```python
from build123d import *

# Parameters (mm, degrees)
CLAMP_START                     = -20.15
CLAMP_X_BASE_DEPTH              = 37.1
WIRE_START                      = -4.99
WIRE_CHANNEL_X_BASE_Z_5_0_DEPTH = 3.42
WIRE_START_2                    = -4.84
SKETCH3_W                       = 1.6
SKETCH3_H                       = 4.320657937
WIRE_NOTCH_X_BASE_Z_5_0_DEPTH   = 3.12
EAR_START                       = -26.1
SKETCH4_W                       = 4.582851153
SKETCH4_H                       = 2.45
EAR_X_BASE_26_DEPTH             = 5.95
EAR_START_2                     = 16.95
SKETCH5_W                       = 4.582851153
SKETCH5_H                       = 2.45
EAR_X_BASE_17_DEPTH             = 5.95
CUT_EXTRUDE3_START              = -6.55
SKETCH6_R                       = 1.05
CUT_EXTRUDE3_DEPTH              = 2.65
CUT_EXTRUDE4_START              = -5.91
SKETCH7_R                       = 2
CUT_EXTRUDE4_DEPTH              = 1.92
CUT_EXTRUDE5_START              = -5.91
SKETCH8_W                       = 2.082851153
SKETCH8_H                       = 4
CUT_EXTRUDE5_DEPTH              = 1.92
CUT_EXTRUDE6_START              = -5.91
CUT_EXTRUDE6_DEPTH              = 1.92
CUT_EXTRUDE7_START              = -5.91
CUT_EXTRUDE7_DEPTH              = 1.92
BOSS_EXTRUDE4_START             = -4
SKETCH11_W                      = 3.882851153
SKETCH11_H                      = 7.3
BOSS_EXTRUDE4_DEPTH             = 0.75


with BuildPart() as part:
    # Sketch1 → Clamp +X base (new body)
    with BuildSketch(Plane.XY.offset(CLAMP_START)):
        Polygon((13.367148847, -4), (17.397275866, -4), (17.397275866, -8.470102587), (13.367148847, -10.796897507), align=None)
    extrude(amount=CLAMP_X_BASE_DEPTH)

    # Sketch2 → Wire channel +X base Z -5.0 (cut)
    with BuildSketch(Plane.XY.offset(WIRE_START)):
        Polygon((11.102085338, -12.220102587), (19.762339376, -7.220102587), (18.912339376, -5.747859401), (10.252085338, -10.747859401), align=None)
    extrude(amount=WIRE_CHANNEL_X_BASE_Z_5_0_DEPTH, mode=Mode.SUBTRACT)

    # Sketch3 → Wire notch +X base Z -5.0 (cut)
    with BuildSketch(Plane.XY.offset(WIRE_START_2)):
        with Locations((16.897275866, -6.060328969)):
            Rectangle(SKETCH3_W, SKETCH3_H)
    extrude(amount=WIRE_NOTCH_X_BASE_Z_5_0_DEPTH, mode=Mode.SUBTRACT)

    # Sketch4 → Ear +X base -26 (add)
    with BuildSketch(Plane.XY.offset(EAR_START)):
        with Locations((15.658574424, -5.225)):
            Rectangle(SKETCH4_W, SKETCH4_H)
    extrude(amount=EAR_X_BASE_26_DEPTH)

    # Sketch5 → Ear +X base 17 (add)
    with BuildSketch(Plane.XY.offset(EAR_START_2)):
        with Locations((15.658574424, -5.225)):
            Rectangle(SKETCH5_W, SKETCH5_H)
    extrude(amount=EAR_X_BASE_17_DEPTH)

    # Sketch6 → Cut-Extrude3 (cut)
    with BuildSketch(Plane(origin=(0, 0, 0), x_dir=(1, 0, 0), z_dir=(0, 1, 0)).offset(CUT_EXTRUDE3_START)):
        with Locations(Location((15.35, 23.2, 0), (0, 0, 90))):
            Circle(SKETCH6_R)
        with Locations(Location((15.35, -20, 0), (0, 0, 90))):
            Circle(SKETCH6_R)
    extrude(amount=CUT_EXTRUDE3_DEPTH, mode=Mode.SUBTRACT)

    # Sketch7 → Cut-Extrude4 (cut)
    with BuildSketch(Plane(origin=(0, 0, 0), x_dir=(1, 0, 0), z_dir=(0, 1, 0)).offset(CUT_EXTRUDE4_START)):
        with Locations((15.35, 23.2)):
            Circle(SKETCH7_R)
        with Locations((15.35, -20)):
            Circle(SKETCH7_R)
    extrude(amount=CUT_EXTRUDE4_DEPTH, mode=Mode.SUBTRACT)

    # Sketch8 → Cut-Extrude5 (cut)
    with BuildSketch(Plane(origin=(0, 0, 0), x_dir=(1, 0, 0), z_dir=(0, 1, 0)).offset(CUT_EXTRUDE5_START)):
        with Locations((14.308574424, 23.2)):
            Rectangle(SKETCH8_W, SKETCH8_H)
        with Locations((14.308574424, -20)):
            Rectangle(SKETCH8_W, SKETCH8_H)
    extrude(amount=CUT_EXTRUDE5_DEPTH, mode=Mode.SUBTRACT)

    # Sketch9 → Cut-Extrude6 (cut)
    with BuildSketch(Plane(origin=(0, 0, 0), x_dir=(1, 0, 0), z_dir=(0, 1, 0)).offset(CUT_EXTRUDE6_START)):
        Polygon((15.35, 25.2), (16.764213562, 24.614213562), (17.35, 24.028427125), (17.35, 22.371572875), (16.764213562, 21.785786438), (15.35, 21.2), align=None)
    extrude(amount=CUT_EXTRUDE6_DEPTH, mode=Mode.SUBTRACT)

    # Sketch10 → Cut-Extrude7 (cut)
    with BuildSketch(Plane(origin=(0, 0, 0), x_dir=(1, 0, 0), z_dir=(0, 1, 0)).offset(CUT_EXTRUDE7_START)):
        Polygon((15.35, -18), (16.764213562, -18.585786438), (17.35, -19.171572875), (17.35, -20.828427125), (16.764213562, -21.414213562), (15.35, -22), align=None)
    extrude(amount=CUT_EXTRUDE7_DEPTH, mode=Mode.SUBTRACT)

    # Sketch11 → Boss-Extrude4 (add)
    with BuildSketch(Plane(origin=(0, 0, 0), x_dir=(1, 0, 0), z_dir=(0, 1, 0)).offset(BOSS_EXTRUDE4_START)):
        with Locations((15.308574424, 11.55)):
            Rectangle(SKETCH11_W, SKETCH11_H)
    extrude(amount=BOSS_EXTRUDE4_DEPTH)


solid = part.part
```
The model under review builds one solid part; all positions refer to its coordinate system, in mm. A direction names the side the tool comes from. Round coordinates to 2 decimals unless told otherwise and drop trailing zeros. Loops run counter-clockwise (first coordinate to the right, second up) from the corner with the lowest first, then second, coordinate; pieces in that order, holes last. Notation, with made-up numbers: (32.25, 84) -> (39.25, 84) arc R28 cw to (39.25, 108) -> close; hole circle Ø10 at (28.5, 57). An arc over 180 degrees is marked (long way). Answer as a JSON object with one key per item and string values. Group by question number.
1) We need section D-D on z = -13.5. Write out the cut boundary in (x, y).
2) We need section A-A on z = 20. Write out the cut boundary in (x, y).
3) Mouldability with a two-part tool opening along Z and no side actions: class faces 1 (the face through (16, -5, 22.9)), 2 (the face through (17.35, -5, -23)), 3 (the face through (13.367, -7, -2)) as released by +Z, released by -Z, zero draft, split by the parting line, or undercut.
4) We need section C-C on y = -9.75. Write out the cut boundary in (x, z).
5) For line 1 (Z direction, x = 15.15, y = -5); line 2 (X direction, y = -6.1, z = -23.2); line 3 (Z direction, x = 14, y = -9.25), list the stretches that pass through material, from the lowest coordinate up. Write a range as [from, to].
6) For faces 4 (the face through (16.13, -4.97, 18.16)), 5 (the face through (15, -8, 16.95)), 6 (the face through (17, -6.45, -23)), list the 3-axis set-ups (+Z, -Z, +X, -X, +Y, -Y) from which the entire face can be reached by the end or side of a thin tool; tool diameter is ignored.
7) We need section B-B on y = -5.25. Write out the cut boundary in (x, z).
8) For pin 1 Ø1.5 at (y, z) = (-6, -18.5) entering from +X; pin 2 Ø1.5 at (x, y) = (15.5, -8.5) entering from -Z; pin 3 Ø1.2 at (x, y) = (16.5, -8.5) entering from -Z, all flat-tipped, find the tip position at first contact; note any pin that passes through.
Result set:
{
 "1": {"outline": "(13.37, -10.8) -> (17.4, -8.47) -> (17.4, -4) -> (17.25, -4) -> (17.25, -3.25) -> (13.37, -3.25) -> close"},
 "2": {"outline": "(13.37, -6.45) -> (14.3, -6.45) -> (14.3, -5.91) -> (13.37, -5.91) -> close; (16.4, -6.45) -> (17.95, -6.45) -> (17.95, -4) -> (17.35, -4) -> (17.35, -5.91) -> (16.4, -5.91) -> close"},
 "3": {"face 1": "released by +Z", "face 2": "undercut", "face 3": "zero draft"},
 "4": {"outline": "(13.37, -20.15) -> (15.18, -20.15) -> (15.18, -4.99) -> (13.37, -4.99) -> close; (13.37, -1.57) -> (15.18, -1.57) -> (15.18, 16.95) -> (13.37, 16.95) -> close"},
 "5": {"line 1": "[-26.1, -25.2], [-21.2, 18], [22, 22.9]", "line 2": "[13.37, 14.3], [16.4, 17.95]", "line 3": "[-20.15, -4.99], [-1.57, 16.95]"},
 "6": {"face 4": "-X, +Y", "face 5": "+Z, +X, -X, -Y", "face 6": "-Z, +X, -X, -Y"},
 "7": {"outline": "(13.37, -26.1) -> (17.95, -26.1) -> (17.95, -20.15) -> (17.4, -20.15) -> (17.4, -4.84) -> (16.1, -4.84) -> (16.1, -1.72) -> (17.4, -1.72) -> (17.4, 16.95) -> (17.95, 16.95) -> (17.95, 22.9) -> (13.37, 22.9) -> (13.37, 22) -> (15.35, 22) arc R2 cw to (16.76, 21.41) -> (17.35, 20.83) -> (17.35, 19.17) -> (16.76, 18.59) arc R2 cw to (15.35, 18) -> (13.37, 18) -> (13.37, -21.2) -> (15.35, -21.2) arc R2 cw to (16.76, -21.79) -> (17.35, -22.37) -> (17.35, -24.03) -> (16.76, -24.61) arc R2 cw to (15.35, -25.2) -> (13.37, -25.2) -> close"},
 "8": {"pin 1": "x = 17.4", "pin 2": "z = -20.15", "pin 3": "z = -20.15"}
}
